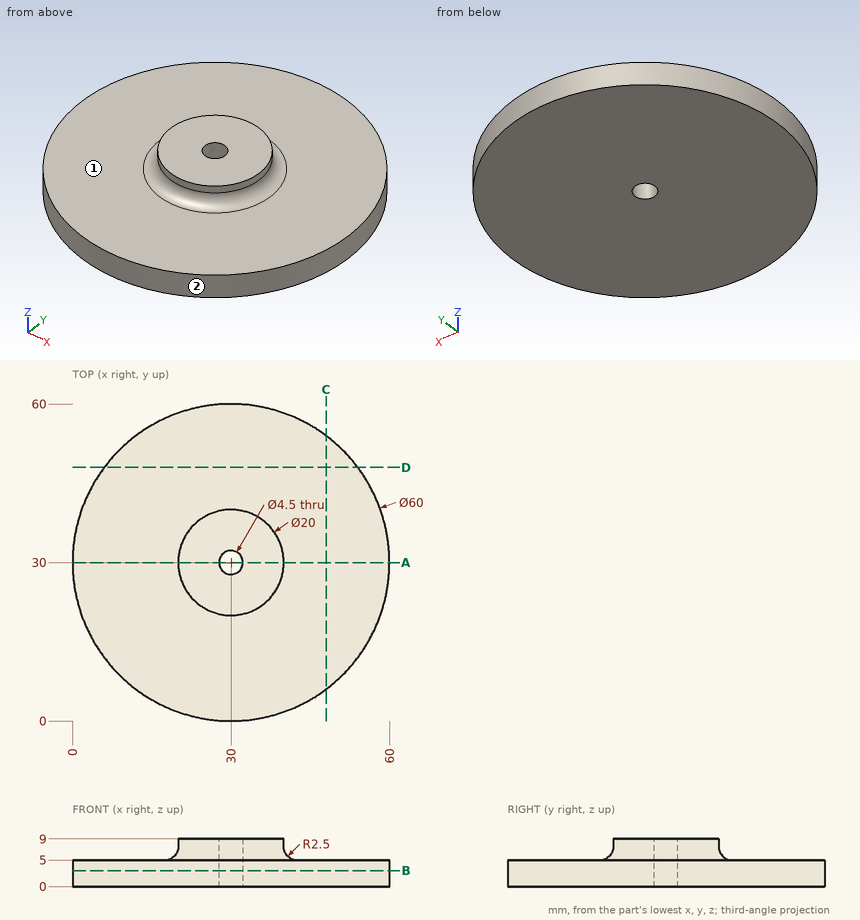
Design review of the part shown in the three views and the two pictorial views. Dimensions are in mm from the part's minimum x, y and z. A direction names the side the tool comes from. Round coordinates to 2 decimals unless told otherwise and drop trailing zeros. Write each loop counter-clockwise with the first axis right and the second up, starting at its lowest first coordinate (ties: lowest second). Pieces come first, ordered by that corner, then holes.
Item 1: Consider section B-B on z = 3. Give the boundary of the cut face in (x, y).
Item 2: Consider section A-A on y = 30. Give the boundary of the cut face in (x, z), and give its area (3 significant figures).
Item 3: Consider section C-C on x = 48. Give the boundary of the cut face in (y, z).
Item 4: For pin 1 Ø1.5 at (x, z) = (16, 5) entering from -Y; pin 2 Ø2 at (x, z) = (11, 4) entering from -Y; pin 3 Ø1 at (x, y) = (51, 47) entering from +Z, all flat-tipped, find the tip position at first contact; note any pin that passes through.
Item 5: Wall thickness on L1, parallel to Y at x = 30, z = 4.5; L2, parallel to Z at x = 56.5, y = 20; L3, parallel to Y at x = 38.5, z = 7: over which ranges is each line inside the solid? List them lowest first.
Item 6: For the marked faces 1 and 2, list the 3-axis set-ups (+Z, -Z, +X, -X, +Y, -Y) from which the entire face can be reached by the end or side of a thin tool; tool diameter is ignored.
Check values:
1. outline: circle Ø60 at (30, 30); hole circle Ø4.5 at (30, 30)
2. outline: (0, 0) - (27.75, 0) - (27.75, 9) - (20, 9) - (20, 7.5) arc R2.5 cw to (17.5, 5) - (0, 5) - close; (32.25, 0) - (60, 0) - (60, 5) - (42.5, 5) arc R2.5 cw to (40, 7.5) - (40, 9) - (32.25, 9) - close
2. area: 342 mm2
3. outline: (6, 0) - (54, 0) - (54, 5) - (6, 5) - close
4. pin 1: stops at y = 3.08
4. pin 2: stops at y = 6
4. pin 3: stops at z = 5
5. L1: y = 0 to 27.75, 32.25 to 60
5. L2: z = 0 to 5
5. L3: y = 24.64 to 35.36
6. face 1: +Z
6. face 2: +Z, -Z
